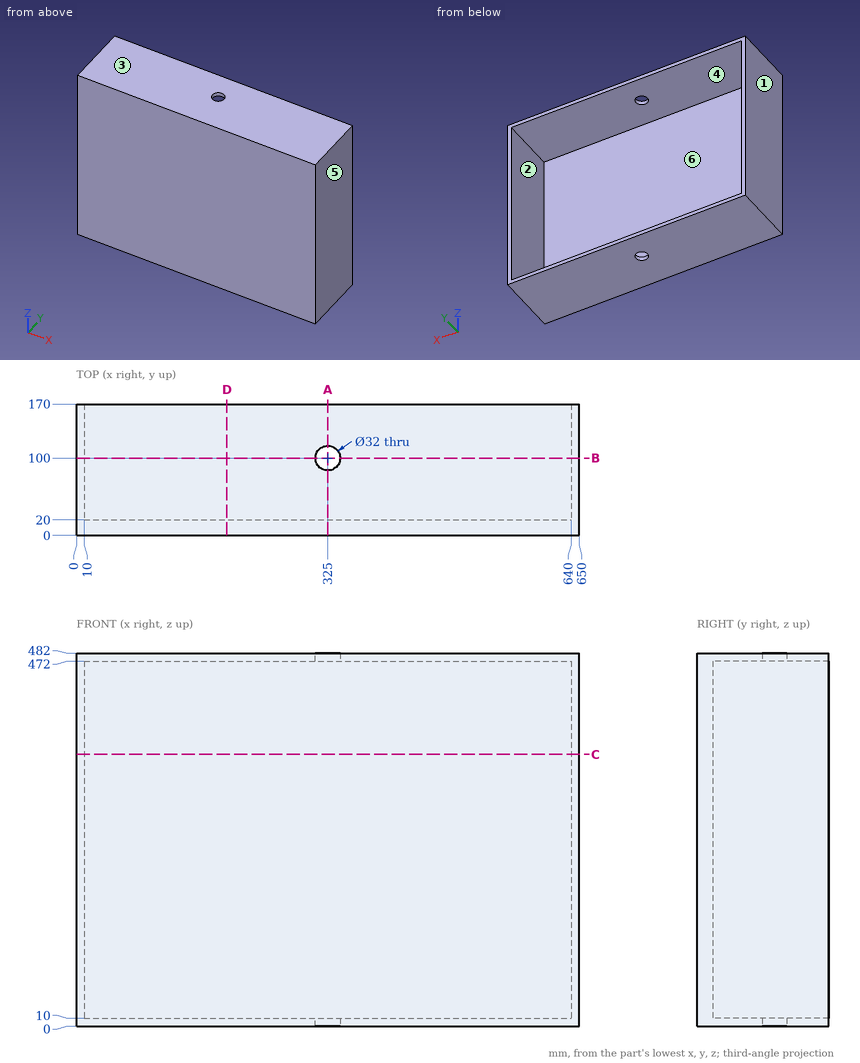
Geometry: see drawing. Coordinates: mm, zero at the bounding-box minimum. A direction names the side the tool comes from. Round coordinates to 2 decimals unless told otherwise and drop trailing zeros. Write each loop counter-clockwise with the first axis right and the second up, starting at its lowest first coordinate (ties: lowest second). Pieces come first, ordered by that corner, then holes. Notation, with made-up numbers: (-28, 74.25) -> (14, 74.25) arc R10 ccw to (14, 82.25) -> close; hole circle Ø2 at (37.25, 30.25). An arc over 180 degrees is marked (long way). Answer as CSV lines item,"result".
1. Section A-A (x = 325). Return the cut outline in (y, z).
Geometry says:
outline,"(0, 0) -> (84, 0) -> (84, 10) -> (20, 10) -> (20, 472) -> (84, 472) -> (84, 482) -> (0, 482) -> close; (116, 0) -> (170, 0) -> (170, 10) -> (116, 10) -> close; (116, 472) -> (170, 472) -> (170, 482) -> (116, 482) -> close"
2. Section D-D (x = 194.5). Return the cut outline in (y, z), plus the area to 3 significant figures.
Geometry says:
outline,"(0, 0) -> (170, 0) -> (170, 10) -> (20, 10) -> (20, 472) -> (170, 472) -> (170, 482) -> (0, 482) -> close"
area,"12,600 mm^2"
3. Mould query, pull axis Z, two halves, no side actions, for the marked faces 3, 4, 5 and 6. Classes: +Z half, -Z half, draft (parallel to the pull), parting line (faces both ways), or undercut.
Geometry says:
face 3,"+Z half"
face 4,"undercut"
face 5,"draft"
face 6,"undercut"
4. Section C-C (z = 351.5). Return the cut outline in (x, y), plus the area to 3 significant figures.
Geometry says:
outline,"(0, 0) -> (650, 0) -> (650, 170) -> (640, 170) -> (640, 20) -> (10, 20) -> (10, 170) -> (0, 170) -> close"
area,"16,000 mm^2"
5. Reachability of the marked faces 1 and 2 from +Z, -Z, +X, -X, +Y, -Y: full face, straight path, thin tool, end or side. Return the list, or none.
Geometry says:
face 1,"+Z, -Z, -X, +Y, -Y"
face 2,"+Y"
6. Ray query, L1, parallel to Z at x = 457, y = 102.5; L2, parallel to Y at x = 325, z = 479; L3, parallel to X at y = 40.5, z = 72. Return the intervals inside material, ascending. Write a range as [from, to].
Geometry says:
L1,"z = [0, 10], [472, 482]"
L2,"y = [0, 84], [116, 170]"
L3,"x = [0, 10], [640, 650]"
7. Contact query for a flat-ended pin moving along its axis: P1, Ø5, axis at y = 98.5, z = 87, coming from the -X side. Output: stop coordinate, or through.
Geometry says:
P1,"stops at x = 0"
8. Section B-B (y = 100). Return the cut outline in (x, z), plus the area to 3 significant figures.
Geometry says:
outline,"(0, 0) -> (309, 0) -> (309, 10) -> (10, 10) -> (10, 472) -> (309, 472) -> (309, 482) -> (0, 482) -> close; (341, 0) -> (650, 0) -> (650, 482) -> (341, 482) -> (341, 472) -> (640, 472) -> (640, 10) -> (341, 10) -> close"
area,"21,600 mm^2"
